Geometry: final body of the model. Coordinates: model frame, mm. A direction names the side the tool comes from. Give positions to 0.01 mm unless a question says otherwise; leave off trailing zeros. Write each loop counter-clockwise with the first axis right and the second up, starting at its lowest first coordinate (ties: lowest second). Pieces come first, ordered by that corner, then holes. Notation, with made-up numbers: (18, -27.75) -> (48, -27.75) arc R24 cw to (48, 11.25) -> close; hole circle Ø1 at (36, 10). An arc over 180 degrees is marked (long way). Answer as a JSON object with one key per item and string values.
Autodesk Inventor part; units mm, degrees
ref_plane "YZ Plane" through (0, 0, 0) normal (1, 0, 0) x (0, 1, 0)
ref_plane "XZ Plane" through (0, 0, 0) normal (0, 1, 0) x (-1, 0, 0)
ref_plane "XY Plane" through (0, 0, 0) normal (0, 0, 1) x (1, 0, 0)
sketch "Sketch1" plane through (0, 0, 0) normal (0, 0, 1) x (1, 0, 0)
  circle A0 centre (21.3984, 18.434) radius 21
  circle A1 centre (21.3984, 18.434) radius 7.5
  point P0 (0, 0)
  dimension "d0" = 42
  dimension "d1" = 15
extrude "Extrusion1" add sketch "Sketch1" along normal blind 30
sketch "Sketch2" plane through (21.3984, 18.434, 30) normal (0, 0, 1) x (1, 0, 0)
  circle A0 centre (0, 0) radius 21
  line L0 (-10.5244, 16.6581) -> (-10.5244, 45.6581)
  line L1 (-10.5244, 45.6581) -> (-3.5244, 45.6581)
  line L2 (-3.5244, 45.6581) -> (-3.5244, 16.6581)
  line L3 (-3.5244, 16.6581) -> (3.4756, 16.6581)
  line L4 (3.4756, 16.6581) -> (3.4756, 45.6581)
  line L5 (3.4756, 45.6581) -> (10.4756, 45.6581)
  line L6 (10.4756, 45.6581) -> (10.4756, 16.6581)
  line L7 (10.4756, 16.6581) -> (-10.5244, 16.6581)
  line L8 (-9.1375, -17.4281) -> (-34.2309, -31.9649)
  line L9 (-34.2309, -31.9649) -> (-37.7398, -25.9078)
  line L10 (-37.7398, -25.9078) -> (-12.6464, -11.371)
  line L11 (-12.6464, -11.371) -> (-16.1552, -5.314)
  line L12 (-16.1552, -5.314) -> (-41.2487, -19.8508)
  line L13 (-41.2487, -19.8508) -> (-44.7576, -13.7938)
  line L14 (-44.7576, -13.7938) -> (-19.6641, 0.7431)
  line L15 (-19.6641, 0.7431) -> (-9.1375, -17.4281)
  line L16 (19.6619, 0.8008) -> (44.7979, -13.6624)
  line L17 (44.7979, -13.6624) -> (41.3067, -19.7297)
  line L18 (41.3067, -19.7297) -> (16.1708, -5.2666)
  line L19 (16.1708, -5.2666) -> (12.6797, -11.3339)
  line L20 (12.6797, -11.3339) -> (37.8156, -25.797)
  line L21 (37.8156, -25.797) -> (34.3245, -31.8643)
  line L22 (34.3245, -31.8643) -> (9.1886, -17.4012)
  line L23 (9.1886, -17.4012) -> (19.6619, 0.8008)
  point P0 (-21.3984, -18.434)
  point P1 (14.4252, -8.3002)
  point P2 (16.1708, -5.2666)
  point P3 (12.6797, -11.3339)
  point P4 (-16.1552, -5.314)
  point P5 (-3.5244, 16.6581)
  point P6 (3.4756, 16.6581)
  dimension "d6" = 29
  dimension "d7" = 7
  dimension "d8" = 29
  dimension "d9" = 7
  dimension "d10" = 29
  dimension "d11" = 7
  dimension "d12" = 29
  dimension "d13" = 45.6581
  dimension "d14" = 3.5244
  dimension "d15" = 29
  dimension "d16" = 7
  dimension "d17" = 29
  dimension "d18" = 7
  dimension "d19" = 29
  dimension "d20" = 7
  dimension "d21" = 29
  dimension "d26" = 29
  dimension "d27" = 7
  dimension "d28" = 29
  dimension "d29" = 7
  dimension "d30" = 29
  dimension "d31" = 7
  dimension "d32" = 29
  dimension "d33" = 29.916
  dimension "d34" = 30.084
  dimension "d35" = 34.3223
  dimension "d36" = 59.3205
  dimension "d37" = 44.8708
  dimension "d38" = 30.163
extrude "Extrusion2" add sketch "Sketch2" against normal blind 30 contours A0 L18 L23 L16 | A0 L16 L17 L18 | L6 L7 L4 A0 | A0 L4 L5 L6 | L20 L21 L22 A0 | A0 L22 L23 L20 | L2 L7 L0 A0 | A0 L0 L1 L2 | L8 L9 L10 A0 | A0 L10 L15 L8 | L14 L15 L12 A0 | A0 L12 L13 L14
properties part number "Rotor" material "Iron, Gray"
Q1. Mould query, pull axis Y, two halves, no side actions, for faces 4 (the flat face through (52.049, 4.836, 15.21)), 5 (the flat face through (15, 14, 0)), 6 (the flat face through (64.475, 1.78, 15.21)). Classes: pulls with the +Y half, pulls with the -Y half, needs draft (parallel to the pull), parting line crosses it, or undercut.
Values:
{"face 4": "undercut", "face 5": "needs draft", "face 6": "pulls with the -Y half"}
Q2. First-contact query: P1, Ø13.5, axis at y = 55.5, z = 9.5, coming from the +X side; P2, Ø12.5, axis at y = 46, z = 19, coming from the -X side; P3, Ø4, axis at x = 35, y = 44, coming from the +Z side; P4, Ø6, axis at y = 21, z = 18.5, coming from the -X side. Flat tips, straight axial feed; report the tip coordinate or a pass-through.
Values:
{"P1": "x = 31.87", "P2": "x = 10.87", "P3": "through", "P4": "x = -0.3"}
Q3. Cut plane B-B (x = 49). Return the cut outline in (y, z).
Values:
{"outline": "(-9.56, 0) -> (-1.49, 0) -> (-1.49, 30) -> (-9.56, 30) -> close; (6.59, 0) -> (14.67, 0) -> (14.67, 30) -> (6.59, 30) -> close"}
Q4. Cut plane C-C (y = 7.5). Return the cut outline in (x, z), and give its area (3 significant figures).
Values:
{"outline": "(-18.42, 0) -> (-4.46, 0) -> (-4.46, 30) -> (-18.42, 30) -> close; (3.47, 0) -> (39.33, 0) -> (39.33, 30) -> (3.47, 30) -> close; (47.42, 0) -> (61.45, 0) -> (61.45, 30) -> (47.42, 30) -> close", "area": "1,920 mm²"}
Q5. Cut plane A-A (y = 45.5). Return the cut outline in (x, z), and give its area (3 significant figures).
Values:
{"outline": "(10.87, 0) -> (17.87, 0) -> (17.87, 30) -> (10.87, 30) -> close; (24.87, 0) -> (31.87, 0) -> (31.87, 30) -> (24.87, 30) -> close", "area": "420 mm²"}
Q6. Set-up query: faces 1 (the flat face through (17.874, 52, 15)), 2 (the flat face through (-0.787, -6.553, 15.21)), 3 (the flat face through (48.26, -1.06, 15.21)). Return all of +Z, -Z, +X, -X, +Y, -Y with unobstructed straight access to the full face (end or side cutting, diameter ignored); none if empty.
Values:
{"face 1": "+Z, -Z, +Y", "face 2": "+Z, -Z, -Y", "face 3": "+Z, -Z"}
Q7. Material intervals for L1, parallel to X at y = 59, z = 18.75; L2, parallel to Y at x = 22, z = 8; L3, parallel to X at y = 3.5, z = 20, sorted ascending. Write a range as from..to.
Values:
{"L1": "10.87..17.87, 24.87..31.87", "L2": "-2.56..10.96, 25.91..39.43", "L3": "-22.7..-11.36, 2.6..40.33, 54.37..65.46"}
Q8. Cut plane D-D (z = 8.5). Return the cut outline in (x, y).
Values:
{"outline": "(-23.36, 4.64) -> (-19.85, -1.42) -> (1.73, 11.08) arc R21 ccw to (5.24, 5.03) -> (-16.34, -7.47) -> (-12.83, -13.53) -> (10.93, 0.23) arc R21 ccw to (31.93, 0.26) -> (55.72, -13.43) -> (59.21, -7.36) -> (37.6, 5.07) arc R21 ccw to (41.09, 11.14) -> (62.71, -1.3) -> (66.2, 4.77) -> (42.4, 18.46) arc R21 ccw to (31.87, 36.63) -> (31.87, 64.09) -> (24.87, 64.09) -> (24.87, 39.14) arc R21 ccw to (17.87, 39.14) -> (17.87, 64.09) -> (10.87, 64.09) -> (10.87, 36.61) arc R21 ccw to (0.4, 18.4) -> close; hole circle Ø15 at (21.4, 18.43)"}
